CAD build for the part. Positions are in the model's coordinates, mm. A direction names the side the tool comes from. Coordinates: 2 decimals unless noted, no trailing zeros. Order: outer loops, then holes, each group sorted by start corner. A loop starts at its lowest first (then second) coordinate and runs counter-clockwise, first axis right, second up. Notation, with made-up numbers: (44.5, -2.5) - (71.5, -2.5) arc R30 ccw to (71.5, 29.5) - close; hole circle Ø11 at (38, 7). An arc over 180 degrees is marked (long way). Return JSON: item names as keys, results as strings.
Autodesk Inventor part; units mm, degrees
ref_plane "YZ Plane" through (0, 0, 0) normal (1, 0, 0) x (0, 1, 0)
ref_plane "XZ Plane" through (0, 0, 0) normal (0, 1, 0) x (-1, 0, 0)
ref_plane "XY Plane" through (0, 0, 0) normal (0, 0, 1) x (1, 0, 0)
sketch "Sketch1" plane through (0, 0, 0) normal (0, 1, 0) x (-1, 0, 0)
  line L0 (-32, 70.5) -> (-32, 55.5)
  line L1 (-32, -70.5) -> (-32, -55.5)
  arc A0 (11, 30.3335) -> (-32, 55.5) centre (-35.6178, 0) ccw
  arc A1 (-32, -55.5) -> (11, -30.3335) centre (-35.6178, 0) ccw
  line L2 (11, 30.3335) -> (11, -30.3335)
  arc A2 (-32, -70.5) -> (-32, 70.5) centre (-35.5914, 0) ccw
  line L3 (35, 0) -> (11, 0)
  point P0 (0, 0)
  dimension "d1" = 141
  dimension "d2" = 15
  dimension "d3" = 15
  dimension "d7" = 24
extrude "Extrusion1" add sketch "Sketch1" along normal blind 5
properties part number "zablona_oblouk"
Item 1: Band-saw the part on B-B, the plane y = 2.6. List the corners of the cut face in (x, z).
Findings below:
{"outline": "(-11, -30.33) - (-11, 30.33) arc R55.62 cw to (32, 55.5) - (32, 70.5) arc R70.59 ccw to (32, -70.5) - (32, -55.5) arc R55.62 cw to start"}
Item 2: Band-saw the part on C-C, the plane x = 17. List the corners of the cut face in (y, z).
Findings below:
{"outline": "(0, -68.1) - (5, -68.1) - (5, -52.41) - (0, -52.41) - close; (0, 52.41) - (5, 52.41) - (5, 68.1) - (0, 68.1) - close"}
Item 3: Mould opens along Z. For faces 3 (the cylindrical face through (-34.984, 2.465, 1.502)), 4 (the flat face through (32, 2, -63)), 5 (the cylindrical face through (7.213, 2.465, -47.817)) say: released by +Z, released by -Z, zero draft, split by the parting line, or undercut.
Findings below:
{"face 3": "split by the parting line", "face 4": "zero draft", "face 5": "undercut"}
Item 4: Band-saw the part on A-A, the plane x = -6. List the corners of the cut face in (y, z), then the cut area to 3 significant figures.
Findings below:
{"outline": "(0, -57.04) - (5, -57.04) - (5, -36.9) - (0, -36.9) - close; (0, 36.9) - (5, 36.9) - (5, 57.04) - (0, 57.04) - close", "area": "201 mm²"}
Item 5: Drop flat-ended pins along their axis: P1, Ø1, axis at y = 3.5, z = 14, coming from the -X side; P2, Ø1, axis at x = 1.5, y = 1.5, coming from the -Z side; P3, Ø1.5, axis at y = 0.5, z = -34.5, coming from the +X side. Give the stop position or say it passes through.
Findings below:
{"P1": "stops at x = -33.7", "P2": "stops at z = -62.09", "P3": "stops at x = -7.4"}
Item 6: Band-saw the part on D-D, the plane z = 0. List the corners of the cut face in (x, y), then the cut area to 3 significant figures.
Findings below:
{"outline": "(-35, 0) - (-11, 0) - (-11, 5) - (-35, 5) - close", "area": "120 mm²"}
Item 7: Which spindle directions (+Z, -Z, +X, -X, +Y, -Y) get a long thin tool onto all of the face, cutting with end or side? Do faces 1 (the cylindrical face through (7.837, 2.465, 48.183)), 2 (the flat face through (-11.3, 5, -4.9)). Say none if no direction does.
Findings below:
{"face 1": "+X, +Y, -Y", "face 2": "+Z, -Z, +X, -X, +Y"}
Item 8: Wall check: L1, parallel to Z at x = 7.5, y = 2.4; L2, parallel to Z at x = 8, y = 0.6; L3, parallel to X at y = 4.25, z = -61.5. Give the ranges that are in metal, low to high. Write a range as [from, to].
Findings below:
{"L1": "z = [-64.76, -47.99], [47.99, 64.76]", "L2": "z = [-64.98, -48.28], [48.28, 64.98]", "L3": "x = [0.94, 32]"}
